Build history of the part. All positions in model axes, mm. Face numbers are marked on the shaded views. Round coordinates to 2 decimals unless told otherwise and drop trailing zeros. Loops run counter-clockwise (first coordinate to the right, second up) from the corner with the lowest first, then second, coordinate; pieces in that order, holes last.
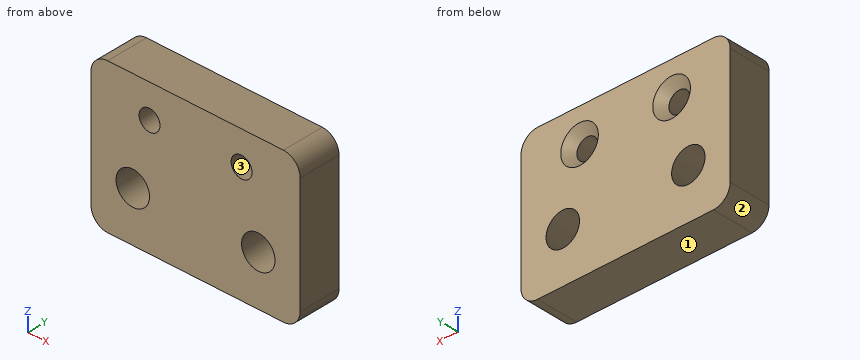
Autodesk Inventor part; units mm, degrees
ref_plane "YZ Plane" through (0, 0, 0) normal (1, 0, 0) x (0, 1, 0)
ref_plane "XZ Plane" through (0, 0, 0) normal (0, 1, 0) x (-1, 0, 0)
ref_plane "XY Plane" through (0, 0, 0) normal (0, 0, 1) x (1, 0, 0)
sketch "Sketch1" plane through (0, 0, 0) normal (0, 1, 0) x (-1, 0, 0)
  line L0 (0, 0) -> (-25, 0)
  line L1 (-25, 0) -> (-25, -18)
  line L2 (-25, -18) -> (0, -18)
  line L3 (0, -18) -> (0, 0)
  circle A0 centre (-7, -4) radius 1.25
  circle A1 centre (-18, -4) radius 1.25
  circle A2 centre (-5, -12) radius 2
  circle A3 centre (-20, -12) radius 2
  dimension "d0" = 25
  dimension "d1" = 18
  dimension "d2" = 2.5
  dimension "d3" = 2.5
  dimension "d4" = 4
  dimension "d5" = 4
  dimension "d6" = 11
  dimension "d7" = 15
  dimension "d8" = 7
  dimension "d9" = 5
  dimension "d10" = 4
  dimension "d11" = 4
  dimension "d12" = 8
extrude "Extrusion1" add sketch "Sketch1" along normal blind 5
fillet "Fillet1" radius 2 4 edges at (0, 2.5, 0) (0, 2.5, -18) (25, 2.5, -18) (25, 2.5, 0)
chamfer "Chamfer1" distance 1 angle 45 1 edges at (8.25, 5, -4)
chamfer "Chamfer2" distance 1 angle 45 1 edges at (19.25, 5, -4)
properties part number "veg_kapcs_tart_csavarral"
(1) Probe line 1 (X direction, y = 3.9, z = -3.5); line 2 (Z direction, x = 5, y = 2.2); line 3 (Z direction, x = 5.5, y = 3.55). List the from-to ranges inside material, lowest first.
Responses:
line 1: x = 0 to 5.85, 8.15 to 16.85, 19.15 to 25
line 2: z = -18 to -14, -10 to 0
line 3: z = -18 to -13.94, -10.06 to 0
(2) Slice it at B-B on y = 0.4. List the corners of the cut face in (x, z), plus the area to 3 significant figures.
Responses:
outline: (0, -16) arc R2 ccw to (2, -18) - (23, -18) arc R2 ccw to (25, -16) - (25, -2) arc R2 ccw to (23, 0) - (2, 0) arc R2 ccw to (0, -2) - close; hole circle Ø4 at (5, -12); hole circle Ø2.5 at (7, -4); hole circle Ø2.5 at (18, -4); hole circle Ø4 at (20, -12)
area: 412 mm2
(3) Slice it at C-C on x = 20.5. List the corners of the cut face in (y, z), plus the area to 3 significant figures.
Responses:
outline: (0, -18) - (5, -18) - (5, -13.94) - (0, -13.94) - close; (0, -10.06) - (5, -10.06) - (5, 0) - (0, 0) - close
area: 70.6 mm2
(4) Pull direction X, two halves, no side cores. Call the marked faces 1, 2 and 3: +X half, -X half, draft (parallel to the pull), parting line (faces both ways), or undercut.
Responses:
face 1: draft
face 2: -X half
face 3: undercut
(5) Slice it at A-A on z = -12. List the corners of the cut face in (x, y).
Responses:
outline: (0, 0) - (3, 0) - (3, 5) - (0, 5) - close; (7, 0) - (18, 0) - (18, 5) - (7, 5) - close; (22, 0) - (25, 0) - (25, 5) - (22, 5) - close
(6) Slice it at D-D on z = -4. List the corners of the cut face in (x, y), plus the area to 3 significant figures.
Responses:
outline: (0, 0) - (5.75, 0) - (5.75, 4) - (4.75, 5) - (0, 5) - close; (8.25, 0) - (16.75, 0) - (16.75, 4) - (15.75, 5) - (9.25, 5) - (8.25, 4) - close; (19.25, 0) - (25, 0) - (25, 5) - (20.25, 5) - (19.25, 4) - close
area: 98.0 mm2
(7) Pin check, flat tip, straight feed: P1, Ø3.5, axis at x = 20, z = -12, coming from the +Y side. Stop position of the tip, or through.
Responses:
P1: passes through
